Source: CAD feature listing. Evaluate the final solid. Frame: model axes, mm. Round coordinates to 2 decimals unless told otherwise and drop trailing zeros. Loops run counter-clockwise (first coordinate to the right, second up) from the corner with the lowest first, then second, coordinate; pieces in that order, holes last.
(1) Section B-B, the plane y = 20.5. Return the cut outline in (x, z), plus the area to 3 significant figures.
(2) Section A-A, the plane x = 0. Return the cut outline in (y, z).
(3) Section C-C, the plane y = 28.5. Return the cut outline in (x, z), plus the area to 3 significant figures.
(4) First-contact query: pin 1 Ø1 at (y, z) = (29.5, 1) entering from +X; pin 2 Ø1 at (x, z) = (20.5, 0.5) entering from -Y; pin 3 Ø2 at (x, y) = (-13.5, 28) entering from +Z; pin 4 Ø3 at (x, y) = (-13.5, 1) entering from +Z. Flat tips, straight axial feed; report the tip coordinate or a pass-through.
(5) Section D-D, the plane z = 0.5. Count the separate pieces of the cut face and the enclosed holes in it, plus the area to 3 significant figures.
(6) Material intervals for probe 1 along Y at (x, z) = (-13, 0.8); probe 2 along X at (y, z) = (20, 1.05); probe 3 along Y at (x, z) = (-14, 1.2), sorted ascending.
Autodesk Inventor part; units mm, degrees
ref_plane "YZ Plane" through (0, 0, 0) normal (1, 0, 0) x (0, 1, 0)
ref_plane "XZ Plane" through (0, 0, 0) normal (0, 1, 0) x (-1, 0, 0)
ref_plane "XY Plane" through (0, 0, 0) normal (0, 0, 1) x (1, 0, 0)
sketch "スケッチ1" plane through (0, 0, 0) normal (0, 0, 1) x (1, 0, 0)
  circle A0 centre (0, 0) radius 10.5 construction
  circle A1 centre (-13.5, 1) radius 1.35
  line L0 (-13.5, 28) -> (13.5, 28) construction
  line L1 (13.5, 28) -> (13.5, 1) construction
  line L2 (13.5, 1) -> (-13.5, 1) construction
  line L3 (-13.5, 1) -> (-13.5, 28) construction
  circle A2 centre (-13.5, 28) radius 1.35
  circle A3 centre (13.5, 1) radius 1.35
  circle A4 centre (13.5, 28) radius 1.35
  line L4 (-19.75, 30.5) -> (-19.75, 27.6)
  line L5 (-19.75, 30.5) -> (19.75, 30.5)
  line L6 (19.75, 30.5) -> (19.75, 27.6)
  line L7 (-19.75, 1.4) -> (-19.75, -1.5)
  line L8 (-19.75, -1.5) -> (-10.6448, -1.5)
  line L9 (19.75, 1.4) -> (19.75, -1.5)
  line L10 (19.75, -1.5) -> (10.6448, -1.5)
  line L11 (-19.75, 25.5) -> (-21.75, 25.5)
  line L12 (-21.75, 25.5) -> (-21.75, 3.5)
  line L13 (-21.75, 3.5) -> (-19.75, 3.5)
  arc A5 (-19.75, 25.5) -> (-19.75, 27.6) centre (-19.75, 26.55) ccw
  arc A6 (-19.75, 1.4) -> (-19.75, 3.5) centre (-19.75, 2.45) ccw
  line L14 (19.75, 25.5) -> (21.75, 25.5)
  line L15 (21.75, 25.5) -> (21.75, 3.5)
  line L16 (21.75, 3.5) -> (19.75, 3.5)
  arc A7 (19.75, 27.6) -> (19.75, 25.5) centre (19.75, 26.55) ccw
  line L17 (0, 28) -> (0, 0) construction
  arc A8 (19.75, 3.5) -> (19.75, 1.4) centre (19.75, 2.45) ccw
  line L18 (-13.5, 14.5) -> (-21.75, 14.5) construction
  arc A9 (10.6448, -1.5) -> (-10.6448, -1.5) centre (0, 0) ccw
  point P0 (0, 30.5)
  dimension "d8" = 21
  dimension "d10" = 27
  dimension "d12" = 1
  dimension "d13" = 2.7
  dimension "d38" = 27
  dimension "d44" = 27
  dimension "d47" = 1.05
  dimension "d48" = 39.5
  dimension "d49" = 2
  dimension "d50" = 5
  dimension "d51" = 32
  dimension "d52" = 5
  dimension "d53" = 10.75
extrude "押し出し1" add sketch "スケッチ1" along normal blind 2
sketch "スケッチ2" plane through (0, 0, 2) normal (0, 0, 1) x (1, 0, 0)
  circle A0 centre (13.5, 28) radius 1.35
  circle A1 centre (-13.5, 28) radius 1.35
  circle A2 centre (-13.5, 1) radius 1.35
  line L0 (-19.75, 30.5) -> (-19.75, 27.6)
  arc A3 (10.6448, -1.5) -> (-10.6448, -1.5) centre (0, 0) ccw
  line L1 (19.75, 30.5) -> (-19.75, 30.5)
  line L2 (-10.542, 27.5) -> (10.542, 27.5)
  line L3 (-16.75, 25) -> (-16.75, 5)
  line L4 (16.75, 25) -> (16.75, 5)
  line L5 (-16.75, 5) -> (-11.7287, 5)
  line L6 (16.75, 5) -> (11.7287, 5)
  arc A4 (11.7287, 5) -> (-11.7287, 5) centre (0, 0) ccw
  line L7 (-16.75, 25) -> (-13.5, 25)
  arc A5 (-13.5, 25) -> (-10.542, 27.5) centre (-13.5, 28) ccw
  line L8 (16.75, 25) -> (13.5, 25)
  arc A6 (10.542, 27.5) -> (13.5, 25) centre (13.5, 28) ccw
  line L9 (0, 30.5) -> (0, 0) construction
  dimension "d56" = 2
  dimension "d57" = 4
  dimension "d58" = 3
  dimension "d59" = 3
  dimension "d60" = 3
extrude "押し出し2" cut sketch "スケッチ2" against normal blind 10 contours L2 A6 L8 L4 L6 A4 L5 L3 L7 A5
fillet "フィレット1" radius 4 8 edges at (10.542, 27.5, 1) (16.75, 25, 1) (16.75, 5, 1) (11.7287, 5, 1) (-11.7287, 5, 1) (-16.75, 5, 1) (-16.75, 25, 1) (-10.542, 27.5, 1)
fillet "フィレット1" radius 2 2 edges at (-10.6448, -1.5, 1) (10.6448, -1.5, 1)
equation "\"d38\" = d10"
equation "\"d44\" = d10"
equation "\"d50\" = d30"
equation "\"d51\" = d18 + 2 * d30"
equation "\"d52\" = d50"
properties part number "足首_サブフレーム_1_1" material "アルミニウム 2014-T4"
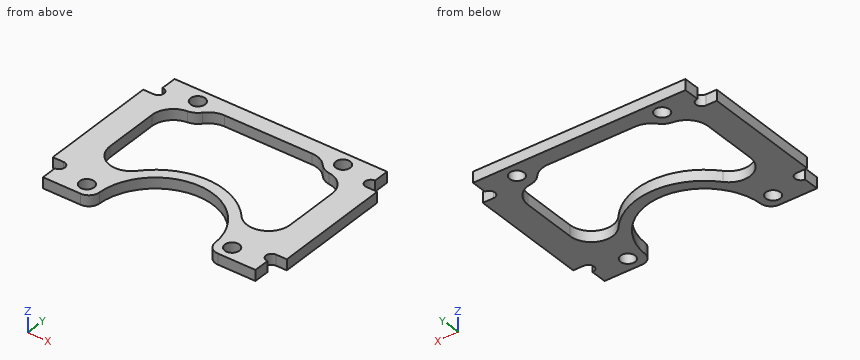
Output values:
1. outline: (-21.75, 0) - (-16.75, 0) - (-16.75, 2) - (-21.75, 2) - close; (16.75, 0) - (21.75, 0) - (21.75, 2) - (16.75, 2) - close
1. area: 20.0 mm2
2. outline: (10.75, 0) - (12.75, 0) - (12.75, 2) - (10.75, 2) - close; (27.5, 0) - (30.5, 0) - (30.5, 2) - (27.5, 2) - close
3. outline: (-19.75, 0) - (-14.75, 0) - (-14.75, 2) - (-19.75, 2) - close; (-12.25, 0) - (12.25, 0) - (12.25, 2) - (-12.25, 2) - close; (14.75, 0) - (19.75, 0) - (19.75, 2) - (14.75, 2) - close
3. area: 69.0 mm2
4. pin 1: stops at x = 19.75
4. pin 2: stops at y = 3.5
4. pin 3: passes through
4. pin 4: stops at z = 2
5. separate pieces: 1
5. enclosed holes: 5
5. area: 548 mm2
6. probe 1: y = -1.5 to -0.25, 2.25 to 6.87, 25.04 to 26.75, 29.25 to 30.5
6. probe 2: x = -21.75 to -16.75, 16.75 to 21.75
6. probe 3: y = -1.5 to -0.25, 2.25 to 7.06, 24.84 to 26.75, 29.25 to 30.5
